from build123d import *

# Parameters (mm, degrees)
SKETCH1_R           = 11.2
BOSS_EXTRUDE1_DEPTH = 15
SKETCH2_R           = 4.125
CUT_EXTRUDE1_DEPTH  = 38
CUT_EXTRUDE2_DEPTH  = 38


with BuildPart() as part:
    # Sketch1 → Boss-Extrude1 (new body)
    with BuildSketch(Plane.XY):
        with BuildLine():
            Line((0, 15.483636231), (31, 15.483636231))
            Line((31, 15.483636231), (31, -15.483636231))
            Line((31, -15.483636231), (0, -15.483636231))
            ThreePointArc((0, -15.483636231), (-15.483636231, 0), (0, 15.483636231))
        make_face()
        Circle(SKETCH1_R, mode=Mode.SUBTRACT)
    extrude(amount=BOSS_EXTRUDE1_DEPTH)

    # Sketch2 → Cut-Extrude1 (cut)
    with BuildSketch(Plane.XZ.offset(15.483636231)):
        with Locations((25.207969837, 9.982935424)):
            Circle(SKETCH2_R)
    extrude(amount=-CUT_EXTRUDE1_DEPTH, mode=Mode.SUBTRACT)

    # Sketch7 → Cut-Extrude2 (cut)
    with BuildSketch(Plane.XY.offset(15)):
        Polygon((25.458117285, 4.5), (13.708117285, 4.5), (13.708117285, -4.5), (31, -4.5), (31, 4.5), align=None)
    extrude(amount=-CUT_EXTRUDE2_DEPTH, mode=Mode.SUBTRACT)


solid = part.part
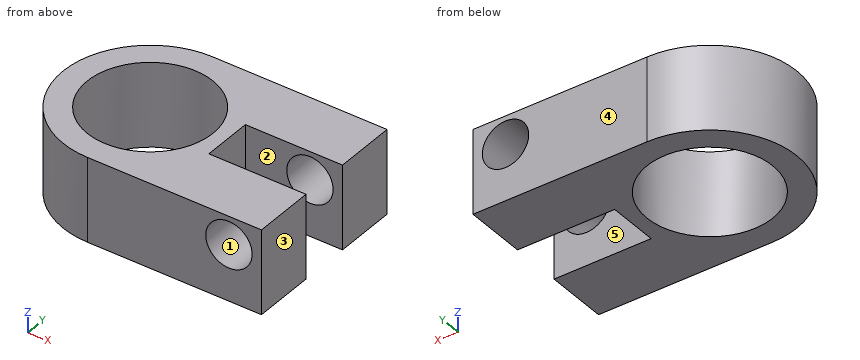
Here's how the part is built. I have some questions about the finished solid (model axes, mm). Face numbers are marked on the shaded views. A direction names the side the tool comes from. Round coordinates to 2 decimals unless told otherwise and drop trailing zeros. Order: outer loops, then holes, each group sorted by start corner. A loop starts at its lowest first (then second) coordinate and runs counter-clockwise, first axis right, second up. Notation, with made-up numbers: (-13, 3.5) -> (18, 3.5) arc R21 ccw to (18, 41.5) -> close; hole circle Ø11 at (69.25, 83.5). An arc over 180 degrees is marked (long way). Use CSV: the item, a comma, the result in double quotes.
1. Thinking about a two-plate mould opening in Y: for the marked faces 3, 4 and 5, which applies, pulls with the +Y half, pulls with the -Y half, needs draft (parallel to the pull), parting line crosses it, or undercut?
Recorded:
face 3,"needs draft"
face 4,"pulls with the +Y half"
face 5,"undercut"
2. I'm going to push flat-ended pins straight in: P1, Ø6, axis at x = 5.5, y = 0.5, coming from the +Z side; P2, Ø2, axis at x = -4, z = 3.5, coming from the +Y side. Where does each tip first touch, or does it pass through?
Recorded:
P1,"passes through"
P2,"stops at y = 15.19"
3. Which directions (+Z, -Z, +X, -X, +Y, -Y) give clear straight access to the entire face, cutting with the end or side of a thin tool? Please do the marked faces 1 and 2.
Recorded:
face 1,"+Y, -Y"
face 2,"+Z, -Z, +X"
4. I want a section at C-C on z = 3.25. List the corners of the cut face in (x, y) for me.
Recorded:
outline,"(0, -15.48) -> (31, -15.48) -> (31, -4.5) -> (13.71, -4.5) -> (13.71, 4.5) -> (31, 4.5) -> (31, 15.48) -> (0, 15.48) arc R15.48 ccw to start; hole circle Ø22.4 at (0, 0)"
5. I need wall thicknesses on line 1 along X through (y, z) = (-9, 7); line 2 along X through (y, z) = (9, 11.75); line 3 along Y through (x, z) = (18.5, 13.25). Which ranges of each line are inside material? Lowest first, please.
Recorded:
line 1,"x = -12.6 to -6.67, 6.67 to 22.36, 28.06 to 31"
line 2,"x = -12.6 to -6.67, 6.67 to 21.48, 28.94 to 31"
line 3,"y = -15.48 to -4.5, 4.5 to 15.48"
6. I want a section at B-B on x = 14.5. List the corners of the cut face in (y, z) for me.
Recorded:
outline,"(-15.48, 0) -> (-4.5, 0) -> (-4.5, 15) -> (-15.48, 15) -> close; (4.5, 0) -> (15.48, 0) -> (15.48, 15) -> (4.5, 15) -> close"
7. I want a section at D-D on y = 8. List the corners of the cut face in (x, z) for me (3 decimals).
Recorded:
outline,"(-13.257, 0) -> (-7.838, 0) -> (-7.838, 15) -> (-13.257, 15) -> close; (7.838, 0) -> (31, 0) -> (31, 15) -> (7.838, 15) -> close; hole circle Ø8.25 at (25.208, 9.983)"
8. I want a section at A-A on y = 0. List the corners of the cut face in (x, z) for me.
Recorded:
outline,"(-15.48, 0) -> (-11.2, 0) -> (-11.2, 15) -> (-15.48, 15) -> close; (11.2, 0) -> (13.71, 0) -> (13.71, 15) -> (11.2, 15) -> close"
